Model file for the job. Use its own axes, mm. Face numbers are marked on the shaded views. A direction names the side the tool comes from. Coordinates: 2 decimals unless noted, no trailing zeros. Write each loop counter-clockwise with the first axis right and the second up, starting at its lowest first coordinate (ties: lowest second). Pieces come first, ordered by that corner, then holes. Notation, with made-up numbers: (63, 34.5) - (122, 34.5) arc R20 cw to (122, 63.5) - close; hole circle Ø1 at (80, 1). An arc over 180 degrees is marked (long way). Put each result on its own line as item: value. Start each with the question number.
1. Saw through at A-A, the plane y = 0. Write the cut outline in (x, z), plus the area to 4 significant figures.
2. Saw through at D-D, the plane x = -4. Write the cut outline in (y, z), plus the area to 3 significant figures.
3. Drop flat-ended pins along their axis: P1, Ø6, axis at x = 4, z = 4.5, coming from the +Y side; P2, Ø3, axis at y = -1.5, z = 7, coming from the +X side; P3, Ø7.5, axis at x = 3.5, y = 0.5, coming from the -Z side; P4, Ø1.5, axis at y = -2, z = 8.5, coming from the -X side. Give the stop position or say it passes through.
4. Saw through at C-C, the plane z = 3. Write the cut outline in (x, y).
5. Pull direction Y, two halves, no side cores. Call the marked faces 4, 5 and 6: released by +Y, released by -Y, zero draft, split by the parting line, or undercut.
6. Which spindle directions (+Z, -Z, +X, -X, +Y, -Y) get a long thin tool onto all of the face, cutting with end or side? Do the marked faces 1, 2 and 3. Say none if no direction does.
7. Drill centre lines: L1, parallel to Y at x = 0, z = 7; L2, parallel to Z at x = 1, y = 6.5; L3, parallel to Y at x = -2.75, z = 5.75. Where is each one in solid material? Low to high. Write a range as from..to.
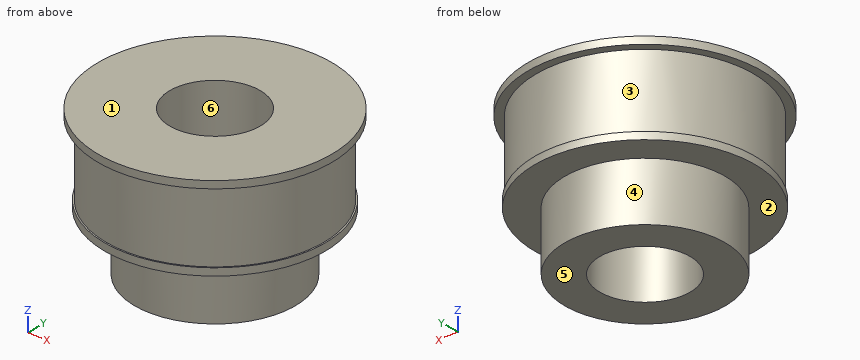
```python
from build123d import *

# Parameters (mm, degrees)
SKETCH_R        = 8
SKETCH_R_2      = 3.1
PAD_DEPTH       = 10
SKETCH001_R     = 15.500543
SKETCH001_R_2   = 7.45
POCKET_DEPTH    = 9.5
SKETCH002_R     = 11.210936
SKETCH002_R_2   = 5.5
POCKET001_DEPTH = 4
SKETCH003_R     = 7.55
SKETCH003_R_2   = 6.749921
PAD001_DEPTH    = 0.5


with BuildPart() as part:
    # Sketch → Pad (new body)
    with BuildSketch(Plane.XY):
        Circle(SKETCH_R)
        Circle(SKETCH_R_2, mode=Mode.SUBTRACT)
    extrude(amount=PAD_DEPTH)

    # Sketch001 (on Face3 of Pad) → Pocket (cut)
    with BuildSketch(Plane(origin=(0, 0, 0), x_dir=(1, 0, 0), z_dir=(0, 0, -1))):
        Circle(SKETCH001_R)
        Circle(SKETCH001_R_2, mode=Mode.SUBTRACT)
    extrude(amount=-POCKET_DEPTH, mode=Mode.SUBTRACT)

    # Sketch002 (on Face6 of Pocket) → Pocket001 (cut)
    with BuildSketch(Plane(origin=(0, 0, 0), x_dir=(1, 0, 0), z_dir=(0, 0, -1))):
        Circle(SKETCH002_R)
        Circle(SKETCH002_R_2, mode=Mode.SUBTRACT)
    extrude(amount=-POCKET001_DEPTH, mode=Mode.SUBTRACT)

    # Sketch003 (on Face6 of Pocket001) → Pad001 (join)
    with BuildSketch(Plane(origin=(0, 0, 4), x_dir=(1, 0, 0), z_dir=(0, 0, -1))):
        Circle(SKETCH003_R)
        Circle(SKETCH003_R_2, mode=Mode.SUBTRACT)
    extrude(amount=-PAD001_DEPTH)


solid = part.part
```
Final values:
1. outline: (-8, 9.5) - (-7.45, 9.5) - (-7.45, 4.5) - (-7.55, 4.5) - (-7.55, 4) - (-5.5, 4) - (-5.5, 0) - (-3.1, 0) - (-3.1, 10) - (-8, 10) - close; (3.1, 0) - (5.5, 0) - (5.5, 4) - (7.55, 4) - (7.55, 4.5) - (7.45, 4.5) - (7.45, 9.5) - (8, 9.5) - (8, 10) - (3.1, 10) - close
1. area: 72.05 mm²
2. outline: (-6.93, 9.5) - (-6.29, 9.5) - (-6.29, 4.5) - (-6.4, 4.5) - (-6.4, 4) - (-3.77, 4) - (-3.77, 0) - (3.77, 0) - (3.77, 4) - (6.4, 4) - (6.4, 4.5) - (6.29, 4.5) - (6.29, 9.5) - (6.93, 9.5) - (6.93, 10) - (-6.93, 10) - close
2. area: 106 mm²
3. P1: stops at y = 7.48
3. P2: stops at x = 7.45
3. P3: stops at z = 0
3. P4: stops at x = -7.34
4. outline: circle Ø11 at (0, 0); hole circle Ø6.2 at (0, 0)
5. face 4: split by the parting line
5. face 5: zero draft
5. face 6: undercut
6. face 1: +Z, +X, -X, +Y, -Y
6. face 2: -Z
6. face 3: none
7. L1: y = -7.45..-3.1, 3.1..7.45
7. L2: z = 4..10
7. L3: y = -6.92..-1.43, 1.43..6.92
